Autodesk Inventor part; units mm, degrees
ref_plane "YZ Plane" through (0, 0, 0) normal (1, 0, 0) x (0, 1, 0)
ref_plane "XZ Plane" through (0, 0, 0) normal (0, 1, 0) x (-1, 0, 0)
ref_plane "XY Plane" through (0, 0, 0) normal (0, 0, 1) x (1, 0, 0)
sketch "Sketch1" plane through (0, 0, 0) normal (0, 0, 1) x (1, 0, 0)
  line L0 (-0.5, -2) -> (0.5, -2)
  line L1 (0.5, 0) -> (0.5, 2)
  line L2 (0.5, 2) -> (-0.5, 2)
  line L3 (-0.5, 2) -> (-0.5, -2)
  line L4 (-0.5, -2) -> (0.5, 2) construction
  line L5 (0.5, -2) -> (-0.5, 2) construction
  line L6 (0.5, -2) -> (5.5, -2)
  line L7 (5.5, -2) -> (5.5, 0)
  line L8 (5.5, 0) -> (0.5, 0)
  point P0 (0, 0)
  dimension "d0" = 1
  dimension "d1" = 4
  dimension "d2" = 5
  dimension "d3" = 14.036
  dimension "d4" = 2
extrude "Extrusion1" add sketch "Sketch1" along normal blind 50
fillet "Fillet1" radius 2 1 edges at (0.5, 0, 25)
fillet "Fillet2" radius 0.5 4 edges at (0.5, 1.9995, 25) (0.5, 2, 25) (5.5, -2, 25) (5.5, 0, 25)
sketch "Sketch2" plane through (-0.5, -2, 0) normal (-1, 0, 0) x (0, 0, 1)
  line L0 (50, 2) -> (0, 2)
  circle A0 centre (2, 2) radius 2
  line L1 (0, 4) -> (50, 4)
  line L2 (50, 4) -> (50, 0)
  circle A1 centre (48, 2) radius 2
  circle A2 centre (25, 2) radius 2
  dimension "d9" = 2
  dimension "d11" = 4
  dimension "d12" = 2
  dimension "d13" = 0
  dimension "d14" = 4
  dimension "d15" = 0
  dimension "d16" = 23
extrude "Extrusion2" add sketch "Sketch2" along normal blind 3 contours A0 L0 | L0 A0 | A2 L0 | L0 A2 | A1 L0 | L0 A1
properties part number "19 bakjes legger"
CAD build for the part. Positions are in the model's coordinates, mm. A direction names the side the tool comes from. Coordinates: 2 decimals unless noted, no trailing zeros. Order: outer loops, then holes, each group sorted by start corner. A loop starts at its lowest first (then second) coordinate and runs counter-clockwise, first axis right, second up.
(1) Saw through at D-D, the plane x = 1.5. Write the cut outline in (y, z).
Solution:
outline: (-2, 0) - (0.27, 0) - (0.27, 50) - (-2, 50) - close
(2) Drill centre lines: L1, parallel to Z at x = -0.75, y = 1.4; L2, parallel to Z at x = -2, y = 0.4; L3, parallel to X at y = 1.55, z = 14.5. Where is each one in solid material? Low to high.
Solution:
L1: z = 0.57 to 3.43, 23.57 to 26.43, 46.57 to 49.43
L2: z = 0.04 to 3.96, 23.04 to 26.96, 46.04 to 49.96
L3: x = -0.5 to 0.55
(3) Saw through at C-C, the plane x = 4.25. Write the cut outline in (y, z), and give its area (3 significant figures).
Solution:
outline: (-2, 0) - (0, 0) - (0, 50) - (-2, 50) - close
area: 100 mm2
(4) Which spindle directions (+Z, -Z, +X, -X, +Y, -Y) get a long thin tool onto all of the face, cutting with end or side? Do faces 5 (the face through (-0.5, -1.6, 49.6)), 6 (the face through (-0.5, -1.5, 0.4)), 7 (the face through (-0.5, 1.6, 0.5)), 8 (the face through (-0.5, 1.6, 49.5)), 9 (the face through (-2, 2, 2)). Say none if no direction does.
Solution:
face 5: +Z, -X, -Y
face 6: -Z, -X, -Y
face 7: -Z, -X, +Y
face 8: +Z, -X, +Y
face 9: -X
(5) Saw through at B-B, the plane y = 0.75. Write the cut outline in (x, z).
Solution:
outline: (-3.5, 0.15) - (-0.5, 0.15) - (-0.5, 0) - (0.94, 0) - (0.94, 50) - (-0.5, 50) - (-0.5, 49.85) - (-3.5, 49.85) - (-3.5, 46.15) - (-0.5, 46.15) - (-0.5, 26.85) - (-3.5, 26.85) - (-3.5, 23.15) - (-0.5, 23.15) - (-0.5, 3.85) - (-3.5, 3.85) - close
(6) Saw through at A-A, the plane x = -1.75. Write the cut outline in (y, z).
Solution:
outline: circle Ø4 at (0, 2); circle Ø4 at (0, 25); circle Ø4 at (0, 48)
(7) Pin check, flat tips, straight feed: pin 1 Ø1.2 at (y, z) = (-0.5, 11) entering from -X; pin 2 Ø3 at (x, z) = (4, 29) entering from +Y; pin 3 Ø2 at (x, z) = (2.5, 24) entering from +Y. Stop position of each tip, or through.
Solution:
pin 1: stops at x = -0.5
pin 2: stops at y = 0
pin 3: stops at y = 0.27
(8) Mould opens along Z. For faces 1 (the face through (-3.5, 0, 2)), 2 (the face through (2, -1, 0)), 3 (the face through (2, -1, 50)), 4 (the face through (-2, 0, 23)) say: released by +Z, released by -Z, zero draft, split by the parting line, or undercut.
Solution:
face 1: zero draft
face 2: released by -Z
face 3: released by +Z
face 4: undercut
